The model under review builds one solid part; all positions refer to its coordinate system, in mm. A direction names the side the tool comes from. Coordinates: 2 decimals unless noted, no trailing zeros. Write each loop counter-clockwise with the first axis right and the second up, starting at its lowest first coordinate (ties: lowest second). Pieces come first, ordered by that corner, then holes. Notation, with made-up numbers: M 4.5,84 L 15.5,84 A33 ccw 15.5,120 Z; hole C 25,32 d5. An arc over 180 degrees is marked long. Answer as a JSON object with one key per item and string values.
```python
from build123d import *

# Parameters (mm, degrees)
BOSS_EXTRUDE1_DEPTH = 1400
SKETCH1_W           = 60
SKETCH1_H           = 45.5
CUT_EXTRUDE1_DEPTH  = 1405.288075859


with BuildPart() as part:
    # Sketch T → Boss-Extrude1 (new body)
    with BuildSketch(Plane(origin=(0, 0, 0), x_dir=(0, 0, -1), z_dir=(1, 0, 0))):
        Polygon((0, 0), (100, 0), (100, -9), (54.5, -9), (54.5, -54), (45.5, -54), (45.5, -9), (0, -9), align=None)
    extrude(amount=BOSS_EXTRUDE1_DEPTH)

    # Sketch1 → Cut-Extrude1 (cut, through all)
    with BuildSketch(Plane(origin=(0, -9, 0), x_dir=(-1, 0, 0), z_dir=(0, -1, 0))):
        with Locations((-330, 22.75)):
            Rectangle(SKETCH1_W, SKETCH1_H)
        with Locations((-540, 22.75)):
            Rectangle(SKETCH1_W, SKETCH1_H)
        with Locations((-1100, 22.75)):
            Rectangle(SKETCH1_W, SKETCH1_H)
        with Locations((-1100, 77.25)):
            Rectangle(SKETCH1_W, SKETCH1_H)
        with Locations((-540, 77.25)):
            Rectangle(SKETCH1_W, SKETCH1_H)
        with Locations((-330, 77.25)):
            Rectangle(SKETCH1_W, SKETCH1_H)
        with Locations((-990, 22.75)):
            Rectangle(SKETCH1_W, SKETCH1_H)
        with Locations((-990, 77.25)):
            Rectangle(SKETCH1_W, SKETCH1_H)
    extrude(amount=-CUT_EXTRUDE1_DEPTH, mode=Mode.SUBTRACT)


solid = part.part
```
(1) Wall thickness on line 1 along X through (y, z) = (-4.5, -7.5); line 2 along Z through (x, y) = (1037, -38.5); line 3 along Y through (x, z) = (386.5, -75): over which ranges is each line inside the solid? List them lowest first. Write a range as from..to.
Results list:
{"line 1": "0..300, 360..510, 570..960, 1020..1070, 1130..1400", "line 2": "-54.5..-45.5", "line 3": "-9..0"}
(2) Add section B-B on x = 1295. Give the boundary of the cut face in (y, z).
Results list:
{"outline": "M -54,-54.5 L -9,-54.5 L -9,-100 L 0,-100 L 0,0 L -9,0 L -9,-45.5 L -54,-45.5 Z"}
(3) Add section C-C on y = -30. Give the boundary of the cut face in (x, z).
Results list:
{"outline": "M 0,-54.5 L 1400,-54.5 L 1400,-45.5 L 0,-45.5 Z"}
(4) Add section A-A on z = -69. Give the boundary of the cut face in (x, y).
Results list:
{"outline": "M 0,-9 L 300,-9 L 300,0 L 0,0 Z; M 360,-9 L 510,-9 L 510,0 L 360,0 Z; M 570,-9 L 960,-9 L 960,0 L 570,0 Z; M 1020,-9 L 1070,-9 L 1070,0 L 1020,0 Z; M 1130,-9 L 1400,-9 L 1400,0 L 1130,0 Z"}
(5) For pin 1 Ø16 at (x, y) = (723, -21.5) entering from +Z; pin 2 Ø1.5 at (x, z) = (1155, -78) entering from +Y; pin 3 Ø13.5 at (x, z) = (1299, -12) entering from -Y; pin 4 Ø1.5 at (x, y) = (503.5, -39) entering from -Z, all flat-tipped, find the tip position at first contact; note any pin that passes through.
Results list:
{"pin 1": "z = -45.5", "pin 2": "y = 0", "pin 3": "y = -9", "pin 4": "z = -54.5"}
(6) For faces 1 (the face through (1263, -9, -23)), 2 (the face through (690, 0, -49)), 3 (the face through (148, -9, -78)), list the 3-axis set-ups (+Z, -Z, +X, -X, +Y, -Y) from which the entire face can be reached by the end or side of a thin tool; tool diameter is ignored.
Results list:
{"face 1": "+Z, +X, -X, -Y", "face 2": "+Z, -Z, +X, -X, +Y", "face 3": "-Z, +X, -X, -Y"}
